Read the model definition and answer for the solid it produces. Units are mm, in the model's axes. Face numbers are marked on the shaded views. A direction names the side the tool comes from. Round coordinates to 2 decimals unless told otherwise and drop trailing zeros. Order: outer loops, then holes, each group sorted by start corner. A loop starts at its lowest first (then second) coordinate and runs counter-clockwise, first axis right, second up. Notation, with made-up numbers: (-5, -28) -> (4, -28) arc R22 ccw to (4, -4) -> close; hole circle Ø10 at (10, 69.5). An arc over 180 degrees is marked (long way). Use a Markdown table: item, result. Add a question column.
1. The mould has two halves that part along X. Classify the marked faces 4, 5 and 6: +X half, -X half, draft (parallel to the pull), parting line (faces both ways), or undercut.
2. Section A-A, the plane y = 38.5 is taken. Give the vertices of the cut face in (x, z).
3. For the marked faces 1, 2 and 3, determine the directions among +Z, -Z, +X, -X, +Y, -Y from which every point of the face is accessible in a straight line to the end or side of a thin tool.
4. Section B-B, the plane y = 15 is taken. Give the vertices of the cut face in (x, z).
5. Given pin 1 (0.8 mm diameter, centred on x = 2, z = -2.5, fed in from +Y); pin 2 (0.5 mm diameter, centred on x = 5, z = -1.5, fed in from +Y); pin 3 (1.5 mm diameter, centred on x = -10.5, z = -1.5, fed in from -Y), each flat-ended and moving along its own axis, determine where each tip first touches the part or whether it passes through.
6. Consider L1, parallel to X at y = 22, z = -0.55; L2, parallel to X at y = 3.5, z = -2.35; L3, parallel to Y at x = -10, z = -1.5. Determine where each line is inside the solid, lowest interval first. Write a range as [from, to].
```python
from build123d import *

# Parameters (mm, degrees)
CUT_EXTRUDE1_DEPTH = 3.5


with BuildPart() as part:
    # Sweep1: sweep along a path in Sketch3
    with BuildLine(Plane(origin=(0, 0, 0), x_dir=(0, 0, -1), z_dir=(1, 0, 0))) as sweep1_path:
        Line((0, 0), (4, 0))
    # Sketch4 → Sweep1 (sweep)
    with BuildSketch(Plane(origin=(0, 0, -4), x_dir=(-1, 0, 0), z_dir=(0, 0, -1))):
        with BuildLine():
            Line((-6.5, 0), (6.5, 0))
            Line((6.5, 0), (6.5, 22))
            ThreePointArc((6.5, 22), (7.378679656, 24.121320344), (9.5, 25))
            Line((9.5, 25), (12.5, 25))
            ThreePointArc((12.5, 25), (13.207106781, 25.292893219), (13.5, 26))
            Line((13.5, 26), (13.5, 34))
            ThreePointArc((13.5, 34), (14.378679656, 36.121320344), (16.5, 37))
            Line((16.5, 37), (21.5, 37))
            Line((21.5, 37), (21.5, 58))
            ThreePointArc((21.5, 58), (21.207106781, 58.707106781), (20.5, 59))
            Line((20.5, 59), (-20.5, 59))
            ThreePointArc((-20.5, 59), (-21.207106781, 58.707106781), (-21.5, 58))
            Line((-21.5, 58), (-21.5, 37))
            Line((-21.5, 37), (-16.5, 37))
            ThreePointArc((-16.5, 37), (-14.378679656, 36.121320344), (-13.5, 34))
            Line((-13.5, 34), (-13.5, 26))
            ThreePointArc((-13.5, 26), (-13.207106781, 25.292893219), (-12.5, 25))
            Line((-12.5, 25), (-9.5, 25))
            ThreePointArc((-9.5, 25), (-7.378679656, 24.121320344), (-6.5, 22))
            Line((-6.5, 22), (-6.5, 0))
        make_face()
    sweep(path=sweep1_path.line)

    # Sketch5 → Cut-Extrude1 (cut)
    with BuildSketch(Plane(origin=(0, 0, -4), x_dir=(-1, 0, 0), z_dir=(0, 0, -1))):
        with BuildLine():
            Line((-1, 0), (1, 0))
            ThreePointArc((1, 0), (1.353553391, 0.146446609), (1.5, 0.5))
            Line((1.5, 0.5), (1.5, 20))
            Line((1.5, 20), (2.5, 20))
            ThreePointArc((2.5, 20), (3.207106781, 20.292893219), (3.5, 21))
            Line((3.5, 21), (3.5, 26))
            ThreePointArc((3.5, 26), (3.792893219, 26.707106781), (4.5, 27))
            Line((4.5, 27), (5.5, 27))
            ThreePointArc((5.5, 27), (6.207106781, 27.292893219), (6.5, 28))
            Line((6.5, 28), (6.5, 58))
            ThreePointArc((6.5, 58), (6.207106781, 58.707106781), (5.5, 59))
            Line((5.5, 59), (-5.5, 59))
            ThreePointArc((-5.5, 59), (-6.207106781, 58.707106781), (-6.5, 58))
            Line((-6.5, 58), (-6.5, 28))
            ThreePointArc((-6.5, 28), (-6.207106781, 27.292893219), (-5.5, 27))
            Line((-5.5, 27), (-4.5, 27))
            ThreePointArc((-4.5, 27), (-3.792893219, 26.707106781), (-3.5, 26))
            Line((-3.5, 26), (-3.5, 21))
            ThreePointArc((-3.5, 21), (-3.207106781, 20.292893219), (-2.5, 20))
            Line((-2.5, 20), (-1.5, 20))
            Line((-1.5, 20), (-1.5, 0.5))
            ThreePointArc((-1.5, 0.5), (-1.353553391, 0.146446609), (-1, 0))
        make_face()
    extrude(amount=-CUT_EXTRUDE1_DEPTH, mode=Mode.SUBTRACT)


solid = part.part
```
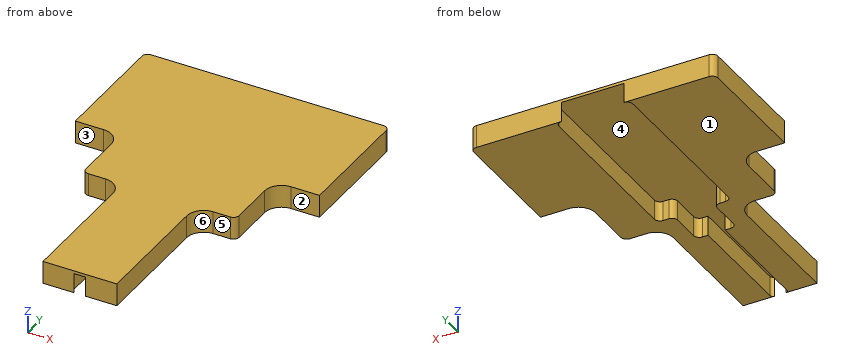
Verdict:
| question | item | result |
|---|---|---|
| 1 | face 4 | undercut |
| 1 | face 5 | draft |
| 1 | face 6 | +X half |
| 2 | outline | (-21.5, -4) -> (-6.5, -4) -> (-6.5, -0.5) -> (6.5, -0.5) -> (6.5, -4) -> (21.5, -4) -> (21.5, 0) -> (-21.5, 0) -> close |
| 3 | face 1 | -Z, +X, -X, +Y, -Y |
| 3 | face 2 | +Z, -Z, +X, -Y |
| 3 | face 3 | +Z, -Z, -X, -Y |
| 4 | outline | (-6.5, -4) -> (-1.5, -4) -> (-1.5, -0.5) -> (1.5, -0.5) -> (1.5, -4) -> (6.5, -4) -> (6.5, 0) -> (-6.5, 0) -> close |
| 5 | pin 1 | stops at y = 20 |
| 5 | pin 2 | stops at y = 27 |
| 5 | pin 3 | stops at y = 25 |
| 6 | L1 | x = [-6.5, -3.5], [3.5, 6.5] |
| 6 | L2 | x = [-6.5, -1.5], [1.5, 6.5] |
| 6 | L3 | y = [25, 59] |
